Autodesk Inventor part; units mm, degrees
ref_plane "Work Plane1" through (-2.7515, 150, 3.6) normal (0, 1, 0) x (1, 0, 0)
ref_plane "YZ Plane" through (0, 0, 0) normal (1, 0, 0) x (0, 1, 0)
ref_plane "XZ Plane" through (0, 0, 0) normal (0, 1, 0) x (-1, 0, 0)
ref_plane "Work Plane1" through (-2.7515, 150, 3.6) normal (0, 1, 0) x (1, 0, 0)
sketch "Sketch1" plane through (-2.7515, 150, 3.6) normal (0, 1, 0) x (1, 0, 0)
  arc A0 (-6.7485, 13.6) -> (-7.2485, 13.1) centre (-6.7485, 13.1) ccw
  line L0 (-7.2485, 13.1) -> (-7.2485, 8.1)
  line L1 (-7.2485, 8.1) -> (-5.7485, 6.6)
  line L2 (-5.7485, 6.6) -> (-5.7485, 9.8)
  line L3 (-5.7485, 9.8) -> (-4.2971, 9.8)
  line L4 (-4.2971, 9.8) -> (-0.8485, 6.3515)
  line L5 (-0.8485, 6.3515) -> (-0.8485, 0.8485)
  line L6 (-0.8485, 0.8485) -> (-4.2971, -2.6)
  line L7 (-4.2971, -2.6) -> (-5.7485, -2.6)
  line L8 (-5.7485, -2.6) -> (-5.7485, 0.6)
  line L9 (-5.7485, 0.6) -> (-7.2485, -0.9)
  line L10 (-7.2485, -0.9) -> (-7.2485, -5.9)
  arc A1 (-7.2485, -5.9) -> (-6.7485, -6.4) centre (-6.7485, -5.9) ccw
  line L11 (-6.7485, -6.4) -> (-1.7485, -6.4)
  line L12 (-1.7485, -6.4) -> (-0.2485, -4.9)
  line L13 (-0.2485, -4.9) -> (-3.4485, -4.9)
  line L14 (-3.4485, -4.9) -> (-3.4485, -3.4485)
  line L15 (-3.4485, -3.4485) -> (0, 0)
  line L16 (0, 0) -> (5.5029, 0)
  line L17 (5.5029, 0) -> (8.9515, -3.4485)
  line L18 (8.9515, -3.4485) -> (8.9515, -4.9)
  line L19 (8.9515, -4.9) -> (5.7515, -4.9)
  line L20 (5.7515, -4.9) -> (7.2515, -6.4)
  line L21 (7.2515, -6.4) -> (12.2515, -6.4)
  arc A2 (12.2515, -6.4) -> (12.7515, -5.9) centre (12.2515, -5.9) ccw
  line L22 (12.7515, -5.9) -> (12.7515, -0.9)
  line L23 (12.7515, -0.9) -> (11.2515, 0.6)
  line L24 (11.2515, 0.6) -> (11.2515, -2.6)
  line L25 (11.2515, -2.6) -> (9.8, -2.6)
  line L26 (9.8, -2.6) -> (6.3515, 0.8485)
  line L27 (6.3515, 0.8485) -> (6.3515, 6.3515)
  line L28 (6.3515, 6.3515) -> (9.8, 9.8)
  line L29 (9.8, 9.8) -> (11.2515, 9.8)
  line L30 (11.2515, 9.8) -> (11.2515, 6.6)
  line L31 (11.2515, 6.6) -> (12.7515, 8.1)
  line L32 (12.7515, 8.1) -> (12.7515, 13.1)
  arc A3 (12.7515, 13.1) -> (12.2515, 13.6) centre (12.2515, 13.1) ccw
  line L33 (12.2515, 13.6) -> (7.2515, 13.6)
  line L34 (7.2515, 13.6) -> (5.7515, 12.1)
  line L35 (5.7515, 12.1) -> (8.9515, 12.1)
  line L36 (8.9515, 12.1) -> (8.9515, 10.6485)
  line L37 (8.9515, 10.6485) -> (5.5029, 7.2)
  line L38 (5.5029, 7.2) -> (0, 7.2)
  line L39 (0, 7.2) -> (-3.4485, 10.6485)
  line L40 (-3.4485, 10.6485) -> (-3.4485, 12.1)
  line L41 (-3.4485, 12.1) -> (-0.2485, 12.1)
  line L42 (-0.2485, 12.1) -> (-1.7485, 13.6)
  line L43 (-1.7485, 13.6) -> (-6.7485, 13.6)
  circle A4 centre (2.7515, 3.6) radius 2
extrude "Extrusion1" add sketch "Sketch1" along normal blind 110
ref_plane "Work Plane2" through (0, 150, -9.5) normal (1, 0, 0) x (0, 0, -1)
ref_plane "Work Plane3" through (-4.5, 150, 0) normal (0, 0, 1) x (1, 0, 0)
properties part number "20x20mmx150mm alminum profile" material "Aluminum 6061"
Build history of the part. All positions in model axes, mm. A direction names the side the tool comes from. Round coordinates to 2 decimals unless told otherwise and drop trailing zeros. Loops run counter-clockwise (first coordinate to the right, second up) from the corner with the lowest first, then second, coordinate; pieces in that order, holes last. Notation, with made-up numbers: (28.5, -6) -> (66.5, -6) arc R33 cw to (66.5, 29) -> close; hole circle Ø9 at (52, -12). An arc over 180 degrees is marked (long way). One line per item, written item: value. Start each with the question number.
Q1. Probe line 1 along X through (y, z) = (226, 0); line 2 along Z through (x, y) = (4.25, 220.5). List the from-to ranges inside material, lowest first.
Q2. Drop flat-ended pins along their axis: pin 1 Ø1.7 at (y, z) = (182.5, 0.5) entering from +X; pin 2 Ø3 at (x, z) = (0, 0) entering from -Y. Give the stop position or say it passes through.
Q3. Cut at B-B on z = 0. List the corners of the cut face in (x, y), plus the area to 3 significant figures.
Q4. Two-plate mould, pull along X, no slides. Class faces 3 (the face through (-10, 204, -7)), 4 (the face through (0, 204, -3.6)), 5 (the face through (7, 204, -10)): released by +X, released by -X, zero draft, split by the parting line, or undercut.
Q5. Cut at A-A on x = 0. List the corners of the cut face in (y, z), plus the area to 3 significant figures.
Q6. 3-axis set-ups, long thin cutter, end or side, ignore diameter. For faces 1 (the face through (-7, 204, -10)), 2 (the face through (-4.5, 204.23, 5.35)): which of +Z, -Z, +X, -X, +Y, -Y reach the whole face in a straight line?
Computed:
1. line 1: -3.6 to -2, 2 to 3.6
1. line 2: -9.75 to -8.5, -5.1 to -3.4, 3.4 to 5.1, 8.5 to 9.75
2. pin 1: x = 3.6
2. pin 2: through
3. outline: (-3.6, 150) -> (-2, 150) -> (-2, 260) -> (-3.6, 260) -> close; (2, 150) -> (3.6, 150) -> (3.6, 260) -> (2, 260) -> close
3. area: 352 mm²
4. face 3: released by -X
4. face 4: undercut
4. face 5: zero draft
5. outline: (150, -3.6) -> (260, -3.6) -> (260, -2) -> (150, -2) -> close; (150, 2) -> (260, 2) -> (260, 3.6) -> (150, 3.6) -> close
5. area: 352 mm²
6. face 1: -Z, +X, -X, +Y, -Y
6. face 2: +Y, -Y
